Model file for the job. Use its own axes, mm. Round coordinates to 2 decimals unless told otherwise and drop trailing zeros. Order: outer loops, then holes, each group sorted by start corner. A loop starts at its lowest first (then second) coordinate and runs counter-clockwise, first axis right, second up. Notation, with made-up numbers: M 84.25,14.25 L 117.25,14.25 A20 ccw 117.25,24.25 Z; hole C 70.5,-15.75 d3. An arc over 180 degrees is marked long. Return JSON: item names as keys, results as strings. Group by question number.
Item 1: Pin check, flat tips, straight feed: pin 1 Ø0.8 at (y, z) = (-4.5, 0) entering from -X; pin 2 Ø1 at (x, z) = (295.5, 0) entering from -Y; pin 3 Ø1.5 at (x, y) = (210.5, 1) entering from -Z; pin 4 Ø5 at (x, y) = (347.5, -2) entering from -Z. Stop position of each tip, or through.
Item 2: Probe line 1 along X through (y, z) = (-3, -0.2); line 2 along X through (y, z) = (0.25, 0.8); line 3 along Z through (x, y) = (47.5, 1.25). List the from-to ranges inside material, lowest first.
Item 3: Slice it at A-A on z = 0. Write the cut outline in (x, y), then the cut area to 3 significant figures.
Item 4: Slice it at B-B on x = 448. Write the cut outline in (y, z).
from build123d import *

# Parameters (mm, degrees)
F0_R      = 0.97
F1_DEPTH  = 525
F2_R      = 0.97
F3_DEPTH  = 6
F4_R      = 0.97
F6_DEPTH  = 14
F7_R      = 0.97
F8_DEPTH  = 6
F11_R     = 0.97
F12_DEPTH = 12


with BuildPart() as f1:
    # F0 (on Right) → F1 (new body)
    with BuildSketch(Plane.YZ):
        Circle(F0_R)
    extrude(amount=F1_DEPTH)

    # F2 (on Front) → F3 (join)
    with BuildSketch(Plane.XZ):
        Circle(F2_R)
    extrude(amount=F3_DEPTH)


with BuildPart() as f1_1:
    # F5: moved
    add(f1.part.moved(Location((0, 2, 0))))

    # F4 (on Right) → F6 (join)
    with BuildSketch(Plane.YZ):
        with Locations((-4.0174978785, 0)):
            Circle(F4_R)
    extrude(amount=F6_DEPTH)



with BuildPart() as f8:
    # F7 (on Front) → F8 (new body)
    with BuildSketch(Plane.XZ):
        with Locations((524.2725610733, 0)):
            Circle(F7_R)
    extrude(amount=F8_DEPTH)


with BuildPart() as f8_1:
    # F9: moved
    add(f8.part.moved(Location((0, 8, 0))))


with BuildPart() as f1_2:
    add(f1_1.part)

    add(f8_1.part)  # F12 merges F8
    # F11 (on face) → F12 (join)
    with BuildSketch(Plane.YZ.offset(524.2725610733)):
        with Locations((8.0255521461, 0)):
            Circle(F11_R)
    extrude(amount=-F12_DEPTH)


solid = f1_2.part
Output values:
{
 "1": {"pin 1": "x = 0", "pin 2": "y = 1.03", "pin 3": "z = -0.94", "pin 4": "through"},
 "2": {"line 1": "-0.95 to 0.95", "line 2": "-0.55 to 0.55", "line 3": "-0.62 to 0.62"},
 "3": {"outline": "M -0.97,-4 L 0,-4 L 0,-4.99 L 14,-4.99 L 14,-3.05 L 0.97,-3.05 L 0.97,1.03 L 525,1.03 L 525,2 L 525.24,2 L 525.24,8 L 524.27,8 L 524.27,9 L 512.27,9 L 512.27,7.06 L 523.3,7.06 L 523.3,2.97 L 0,2.97 L 0,2 L -0.97,2 Z", "area": "1,090 mm²"},
 "4": {"outline": "C 2,0 d1.94"}
}
